Autodesk Inventor part; units mm, degrees
ref_plane "工作平面1" through (10, 19, 0) normal (-0.4554, -0.6295, -0.6295) x (0.8102, 0, -0.5861)
ref_plane "YZ Plane" through (0, 0, 0) normal (1, 0, 0) x (0, 1, 0)
ref_plane "XZ Plane" through (0, 0, 0) normal (0, 1, 0) x (-1, 0, 0)
sketch "草圖1" plane through (0, 0, 0) normal (0, 1, 0) x (-1, 0, 0)
  line L0 (0, 0) -> (-57, 0)
  line L1 (-57, 0) -> (-57, -44)
  line L2 (-57, -44) -> (0, -44)
  line L3 (0, -44) -> (0, 0)
  dimension "d0" = 57
  dimension "d1" = 44
extrude "擠出1" add sketch "草圖1" along normal mid plane 38
sketch "草圖2" plane through (0, 19, 0) normal (0, 1, 0) x (1, 0, 0)
  line L0 (0, 0) -> (57, 0)
  line L1 (10, 0) -> (57, 14)
  line L2 (57, 0) -> (57, 44)
  dimension "d4" = 10
  dimension "d5" = 30
extrude "擠出2" cut sketch "草圖2" against normal blind 40
sketch "草圖3" plane through (57, -19, -44) normal (1, 0, 0) x (0, 0, -1)
  line L0 (-30, 18) -> (-10, 38)
  line L1 (0, 38) -> (-44, 38)
  line L2 (-30, 38) -> (-30, 0)
  point P0 (-44, 19)
  dimension "d8" = 20
  dimension "d9" = 20
ref_plane "工作平面1" through (10, 19, 0) normal (-0.4554, -0.6295, -0.6295) x (0.8102, 0, -0.5861)
sketch "草圖4" plane through (10, 19, 0) normal (-0.4554, -0.6295, -0.6295) x (0.8102, 0, -0.5861)
  line L0 (-15.1543, -12.3218) -> (93.717, -12.3218)
  line L1 (93.717, -12.3218) -> (93.717, 28.8166)
  line L2 (93.717, 28.8166) -> (-15.1543, 28.8166)
  line L3 (-15.1543, 28.8166) -> (-15.1543, -12.3218)
  point P0 (-8.1022, 11.0728)
extrude "擠出3" cut sketch "草圖4" against normal blind 40
mirror "鏡射1" about plane through (0, 0, 0) normal (0, 1, 0) of "擠出3"
properties part number "42"
Input: part model. Units: mm. Frame: model coordinates. Round coordinates to 2 decimals unless told otherwise and drop trailing zeros. Loops run counter-clockwise (first coordinate to the right, second up) from the corner with the lowest first, then second, coordinate; pieces in that order, holes last. Notation, with made-up numbers: (-23, 80.5) -> (13, 80.5) arc R34 ccw to (13, 118.5) -> close; hole circle Ø4 at (36.5, 10). An arc over 180 degrees is marked (long way). Answer as a JSON object with one key per item and string values. Group by question number.
1) Section query B-B on y = -3.5. Output: boundary loops of the cut face in (x, z).
2) Pin query (flat end, axial travel): pin 1 (6 mm diameter, centred on x = 40.5, z = -9.5, fed in from -Y); pin 2 (10 mm diameter, centred on x = 25, y = 1, fed in from +Z); pin 3 (3 mm diameter, centred on x = 12, y = -6, fed in from +Z). Return the tip coordinate at first contact, or that it passes through.
3) Ray query, L1, parallel to Z at x = 14.5, y = -4; L2, parallel to Z at x = 23.5, y = -8.5; L3, parallel to X at y = -8.5, z = -14. Return the intervals inside material, ascending.
4) Section query A-A on x = 49. Output: boundary loops of the cut face in (y, z).
Reply:
{
 "1": {"outline": "(0, -44) -> (57, -44) -> (57, -18.5) -> (46.42, -10.85) -> (10, 0) -> (0, 0) -> close"},
 "2": {"pin 1": "stops at y = -10.13", "pin 2": "stops at z = -2.98", "pin 3": "stops at z = -0.15"},
 "3": {"L1": "z = -44 to -1.34", "L2": "z = -44 to -4.02", "L3": "x = 0 to 43.86"},
 "4": {"outline": "(-19, -44) -> (19, -44) -> (19, -28.22) -> (2.4, -11.62) -> (-2.4, -11.62) -> (-19, -28.22) -> close"}
}
